Autodesk Inventor part; units mm, degrees
ref_plane "YZ Plane" through (0, 0, 0) normal (1, 0, 0) x (0, 1, 0)
ref_plane "XZ Plane" through (0, 0, 0) normal (0, 1, 0) x (-1, 0, 0)
ref_plane "XY Plane" through (0, 0, 0) normal (0, 0, 1) x (1, 0, 0)
sketch "Sketch1" plane through (0, 0, 0) normal (0, 1, 0) x (-1, 0, 0)
  line L0 (0, 0) -> (0, 3.1115)
  line L1 (0, 3.1115) -> (1.524, 3.1115)
  line L2 (1.524, 3.1115) -> (1.524, 4.4323)
  line L3 (1.524, 4.4323) -> (2.6416, 4.4323)
  line L4 (2.6416, 4.4323) -> (3.683, 3.4265)
  line L5 (3.683, 3.4265) -> (3.683, 0.0102)
  line L6 (7.9375, 0.0102) -> (-3.8699, 0.0102) construction
  line L7 (0, 0.0204) -> (0, -3.0911)
  line L8 (0, -3.0911) -> (1.524, -3.0911)
  line L9 (1.524, -3.0911) -> (1.524, -4.4119)
  line L10 (1.524, -4.4119) -> (2.6416, -4.4119)
  line L11 (2.6416, -4.4119) -> (3.683, -3.4061)
  line L12 (3.683, -3.4061) -> (3.683, 0.0102)
  line L13 (3.683, 3.4265) -> (3.683, -3.4061)
  line L14 (0, -3.0911) -> (0, 3.1115)
  line L15 (0, 3.1115) -> (-1.524, 3.1115)
  line L16 (-1.524, 3.1115) -> (-1.524, 4.4323)
  line L17 (-1.524, 4.4323) -> (-2.6416, 4.4323)
  line L18 (-2.6416, 4.4323) -> (-3.683, 3.4265)
  line L19 (-2.6416, -4.4119) -> (-3.683, -3.4061)
  line L20 (-1.524, -4.4119) -> (-2.6416, -4.4119)
  line L21 (-1.524, -3.0911) -> (-1.524, -4.4119)
  line L22 (0, -3.0911) -> (-1.524, -3.0911)
  line L23 (-3.683, 3.4265) -> (-3.683, -3.4061)
  dimension "d1" = 3.1115
  dimension "d2" = 1.524
  dimension "d3" = 1.3208
  dimension "d4" = 1.1176
  dimension "d5" = 1.4478
  dimension "d6" = 3.4163
  dimension "d7" = 3.683
extrude "Extrusion1" add sketch "Sketch1" along normal blind 33.02
properties part number "double slider"
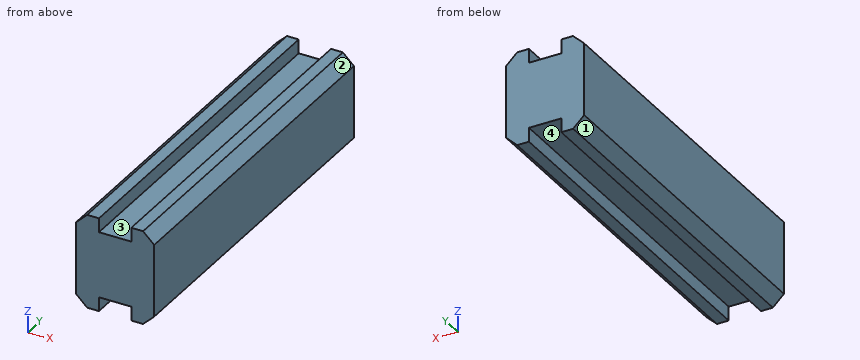
Model file for the job. Use its own axes, mm. Face numbers are marked on the shaded views. Coordinates: 2 decimals unless noted, no trailing zeros. Write each loop counter-clockwise with the first axis right and the second up, starting at its lowest first coordinate (ties: lowest second). Pieces come first, ordered by that corner, then holes. Notation, with made-up numbers: (29.25, -40) -> (82.25, -40) arc R20 cw to (82.25, -6) -> close; hole circle Ø2 at (87.5, 63.5). An arc over 180 degrees is marked (long way). One line per item, written item: value. Start each with the question number.
1) Slice it at A-A on y = 21. Write the cut outline in (x, z).
2) Slice it at B-B on x = 1. Write the cut outline in (y, z), then the cut area to 3 significant figures.
3) Slice it at C-C on x = 3. Write the cut outline in (y, z).
4) Pull direction X, two halves, no side cores. Call the marked faces 1, 2, 3 and 4: +X half, -X half, draft (parallel to the pull), parting line (faces both ways), or undercut.
5) Flat gauge pins, fed straight in: pin 1 Ø0.9 at (x, y) = (-0.5, 12) entering from +Z; pin 2 Ø0.7 at (y, z) = (17, 4) entering from +X. Where does each tip first touch, or does it go through?
6) Probe probe 1 along Z at (x, y) = (-1.25, 12.5); probe 2 along X at (y, z) = (9, 3.75); probe 3 along X at (y, z) = (9.5, 3.5). List the from-to ranges inside material, lowest first.
Answers follow:
1. outline: (-3.68, -3.41) -> (-2.64, -4.41) -> (-1.52, -4.41) -> (-1.52, -3.09) -> (1.52, -3.09) -> (1.52, -4.41) -> (2.64, -4.41) -> (3.68, -3.41) -> (3.68, 3.43) -> (2.64, 4.43) -> (1.52, 4.43) -> (1.52, 3.11) -> (-1.52, 3.11) -> (-1.52, 4.43) -> (-2.64, 4.43) -> (-3.68, 3.43) -> close
2. outline: (0, -3.09) -> (33.02, -3.09) -> (33.02, 3.11) -> (0, 3.11) -> close
2. area: 205 mm2
3. outline: (0, -4.07) -> (33.02, -4.07) -> (33.02, 4.09) -> (0, 4.09) -> close
4. face 1: -X half
4. face 2: +X half
4. face 3: undercut
4. face 4: undercut
5. pin 1: z = 3.11
5. pin 2: x = 3.45
6. probe 1: -3.09 to 3.11
6. probe 2: -3.35 to -1.52, 1.52 to 3.35
6. probe 3: -3.61 to -1.52, 1.52 to 3.61
